Design review of the part built by this model. Coordinates are the model's own, in mm. A direction names the side the tool comes from. Give positions to 0.01 mm unless a question says otherwise; leave off trailing zeros. Loops run counter-clockwise (first coordinate to the right, second up) from the corner with the lowest first, then second, coordinate; pieces in that order, holes last.
Autodesk Inventor part; units mm, degrees
ref_plane "YZ Plane" through (0, 0, 0) normal (1, 0, 0) x (0, 1, 0)
ref_plane "XZ Plane" through (0, 0, 0) normal (0, 1, 0) x (-1, 0, 0)
ref_plane "XY Plane" through (0, 0, 0) normal (0, 0, 1) x (1, 0, 0)
sketch "Esboço1" plane through (0, 0, 0) normal (0, 1, 0) x (-1, 0, 0)
  line L0 (-70, 60) -> (70, 60)
  line L1 (70, 60) -> (70, -60)
  line L2 (70, -60) -> (-70, -60)
  line L3 (-70, -60) -> (-70, 60)
  line L4 (-70, 60) -> (70, -60) construction
  line L5 (70, 60) -> (-70, -60) construction
  point P0 (0, 0)
  dimension "d0" = 140
  dimension "d1" = 120
extrude "Extrusão1" add sketch "Esboço1" along normal blind 1.6
sketch "Esboço2" plane through (0, 1.6, 0) normal (0, 1, 0) x (1, 0, 0)
  line L0 (-94.6357, 0) -> (83.6022, 0)
  line L1 (-70, -37) -> (-52, -37)
  line L2 (-52, 37) -> (-70, 37)
  line L3 (-70, 37) -> (-70, -37)
  line L4 (-70, -37) -> (-52, 37) construction
  line L5 (-52, -37) -> (-70, 37) construction
  line L6 (-70, 60) -> (-70, -60)
  line L7 (-70, 0) -> (-70, 0)
  line L8 (-70, 0) -> (-25, 0)
  circle A0 centre (-25, 0) radius 12.5
  line L9 (-70, -60) -> (70, -60)
  line L10 (-20, -60) -> (-50, -60)
  line L11 (-20, -60) -> (10, -60)
  line L12 (70, 60) -> (-70, 60)
  line L13 (-55, -60) -> (5, -60)
  line L14 (5, -60) -> (5, -45)
  line L15 (-55, -45) -> (-55, -60)
  line L16 (-52, 0) -> (-70, 0)
  line L17 (-56, 25) -> (-48, 25)
  line L18 (-48, 25) -> (-48, -25)
  line L19 (-48, -25) -> (-56, -25)
  line L20 (-56, -25) -> (-56, 25)
  line L21 (-56, 25) -> (-48, -25) construction
  line L22 (-48, 25) -> (-56, -25) construction
  line L23 (-55, 60) -> (5, 60)
  line L24 (5, 60) -> (5, 45)
  line L25 (-55, 45) -> (-55, 60)
  line L26 (-25, 76.0053) -> (-25, -77.5323)
  line L27 (-35, -45) -> (-35, -37)
  line L28 (-35, -37) -> (-15, -37)
  line L29 (-15, -37) -> (-15, -45)
  line L30 (5, -45) -> (-15, -45)
  line L31 (-35, -45) -> (-55, -45)
  line L32 (-35, 45) -> (-35, 37)
  line L33 (-35, 37) -> (-15, 37)
  line L34 (-15, 37) -> (-15, 45)
  line L35 (5, 45) -> (-15, 45)
  line L36 (-35, 45) -> (-55, 45)
  line L37 (-55, -60) -> (5, -45) construction
  line L38 (5, -60) -> (-55, -45) construction
  line L39 (-35, 45) -> (-15, 37) construction
  line L40 (-15, 45) -> (-35, 37) construction
  point P0 (0, 0)
  point P1 (-61, 0)
  point P2 (-25, 41)
  dimension "d4" = 18
  dimension "d5" = 74
  dimension "d6" = 0
  dimension "d7" = 45
  dimension "d8" = 25
  dimension "d28" = 15
  dimension "d30" = 18
  dimension "d31" = 8
  dimension "d32" = 50
  dimension "d35" = 15
  dimension "d36" = 20
  dimension "d38" = 8
  dimension "d40" = 20
  dimension "d41" = 8
  dimension "d42" = 60
  dimension "d43" = 60
extrude "Extrusão4" cut sketch "Esboço2" against normal through all contours L26 A0 L0 | L26 A0 L0 | L0 A0 L26 | L0 A0 L26 | L18 L19 L20 L0 | L0 L20 L17 L18
sketch "Esboço3" plane through (0, 1.6, 0) normal (0, 1, 0) x (1, 0, 0)
  line L0 (44.5, -40) -> (30, -40) construction
  line L1 (30, -40) -> (30, -72.5) construction
  line L2 (30, -72.5) -> (44.5, -72.5) construction
  line L3 (44.5, -72.5) -> (44.5, -40) construction
  line L4 (30, 40) -> (44.5, 40) construction
  line L5 (44.5, 40) -> (44.5, 72.5) construction
  line L6 (44.5, 72.5) -> (30, 72.5) construction
  line L7 (30, 72.5) -> (30, 40) construction
  line L8 (37.25, -40) -> (37.25, -47.2) construction
  circle A0 centre (37.25, -47.2) radius 1.5
  line L9 (37.25, 40) -> (37.25, 47.2) construction
  circle A1 centre (37.25, 47.2) radius 1.5
  line L10 (-70, 60) -> (-70, -60)
  line L11 (52, 14) -> (49.5, 14) construction
  line L12 (49.5, 14) -> (49.5, -14) construction
  line L13 (49.5, -14) -> (52, -14) construction
  line L14 (52, -14) -> (52, 14) construction
  line L15 (52, 14) -> (49.5, -14) construction
  line L16 (49.5, 14) -> (52, -14) construction
  line L17 (54, 16) -> (47.5, 16)
  line L18 (47.5, 16) -> (47.5, -16) construction
  line L19 (47.5, -16) -> (54, -16) construction
  line L20 (54, -16) -> (54, 16)
  line L21 (70, -60) -> (70, 60)
  line L22 (5, -54.0532) -> (28, -36.1915)
  line L23 (28, -36.1915) -> (28, -58)
  line L24 (44.5, -69.5) -> (44.5446, -69.5)
  line L25 (46.5, -58) -> (46.5, -38)
  line L26 (46.5, -38) -> (46.5, -36.8245)
  line L27 (46.5, -58) -> (28, -58)
  line L28 (-70, -60) -> (70, -60)
  line L29 (7, -60) -> (5, -60)
  line L30 (70, 60) -> (-70, 60)
  line L31 (70, 60) -> (7, 60)
  line L32 (5, 54.0532) -> (28, 36.1915)
  line L33 (28, 58) -> (28, 36.1915)
  line L34 (44.5446, 69.5) -> (44.5, 69.5)
  line L35 (46.5, 58) -> (28, 58)
  line L36 (46.5, 36.8245) -> (46.5, 58)
  line L37 (5, 54.0532) -> (5, 60)
  line L38 (5, -54.0532) -> (5, -60)
  line L39 (54, -16) -> (54, -31)
  line L40 (54, -31) -> (46.5, -36.8245)
  line L41 (54, 16) -> (54, 31)
  line L42 (54, 31) -> (46.5, 36.8245)
  point P0 (0, 0)
  dimension "d59" = 14.5
  dimension "d60" = 32.5
  dimension "d63" = 32.5
  dimension "d64" = 14.5
  dimension "d76" = 7.2
  dimension "d77" = 3
  dimension "d78" = 7.2
  dimension "d79" = 3
  dimension "d97" = 2.5
  dimension "d98" = 28
  dimension "d99" = 2
  dimension "d103" = 2
  dimension "d104" = 2
  dimension "d105" = 63
  dimension "d107" = 2
  dimension "d132" = 15
  dimension "d133" = 15
sketch "Esboço4" plane through (0, 1.6, 0) normal (0, 1, 0) x (1, 0, 0)
  line L0 (-70, 60) -> (-70, -60)
  line L1 (-70, 0) -> (-70, -100)
  line L2 (-70, -100) -> (180, -100)
  line L3 (180, -100) -> (180, 100)
  line L4 (180, 100) -> (-70, 100)
  line L5 (-70, 100) -> (-70, -100)
  line L6 (250, 0) -> (-150, 0)
  line L7 (-430, 10) -> (570, 10)
  line L8 (570, 10) -> (570, -10)
  line L9 (570, -10) -> (-430, -10)
  line L10 (-430, -10) -> (-430, 10)
  line L11 (70, -60) -> (70, 60)
  line L12 (-430, 10) -> (570, -10) construction
  line L13 (570, 10) -> (-430, -10) construction
  line L14 (27.5, -90) -> (47.5, -90)
  line L15 (47.5, -90) -> (47.5, -50)
  line L16 (47.5, -50) -> (27.5, -50)
  line L17 (27.5, -50) -> (27.5, -90)
  line L18 (27.5, -90) -> (47.5, -50) construction
  line L19 (47.5, -90) -> (27.5, -50) construction
  line L20 (70, 60) -> (-70, 60)
  line L21 (47.5, 90) -> (27.5, 90)
  line L22 (27.5, 90) -> (27.5, 50)
  line L23 (27.5, 50) -> (47.5, 50)
  line L24 (47.5, 50) -> (47.5, 90)
  line L25 (47.5, 90) -> (27.5, 50) construction
  line L26 (27.5, 90) -> (47.5, 50) construction
  line L27 (0, -100) -> (0, 100) construction
  point P0 (0, 0)
  point P1 (70, 0)
  point P2 (37.5, -70)
  point P3 (37.5, 70)
  dimension "d53" = 100
  dimension "d54" = 250
  dimension "d55" = 200
  dimension "d65" = 1000
  dimension "d66" = 20
  dimension "d68" = 20
  dimension "d69" = 40
  dimension "d70" = 20
  dimension "d71" = 40
  dimension "d72" = 40
  dimension "d73" = 40
  dimension "d80" = 37.5
  dimension "d81" = 37.5
extrude "Extrusão5" cut sketch "Esboço3" against normal through all contours A0 | A1
sketch "Esboço5" plane through (0, 1.6, 0) normal (0, 1, 0) x (1, 0, 0)
  line L0 (70, 60) -> (-70, 60)
  line L1 (-70, 60) -> (-55, 60)
  line L2 (-55, 60) -> (-55, 39)
  line L3 (-55, 39) -> (-70, 39)
  line L4 (-70, 39) -> (-70, 60)
  line L5 (-70, -60) -> (70, -60)
  line L6 (-70, -60) -> (-55, -60)
  line L7 (-55, -60) -> (-55, -39)
  line L8 (-55, -39) -> (-70, -39)
  line L9 (-70, -39) -> (-70, -60)
  line L10 (-70, 60) -> (-70, -60)
  line L11 (-55, 39) -> (-70, 39)
  line L12 (-70, 39) -> (-70, 60)
  line L13 (-70, 60) -> (-55, 60)
  line L14 (-55, 60) -> (-55, 39)
  line L15 (-55, -39) -> (-70, -39)
  line L16 (-70, -39) -> (-70, -60)
  line L17 (-70, -60) -> (-55, -60)
  line L18 (-55, -60) -> (-55, -39)
  point P0 (0, 0)
  dimension "d84" = 15
  dimension "d85" = 21
  dimension "d86" = 15
  dimension "d87" = 21
extrude "Extrusão6" cut sketch "Esboço5" against normal through all
fillet "Arredondamento1" radius 2 10 edges at (-70, 0.8, 39) (-55, 0.8, 39) (-55, 0.8, 60) (-56, 0.8, 25) (-48, 0.8, 25) (-56, 0.8, -25) (-48, 0.8, -25) (-70, 0.8, -39) (-55, 0.8, -39) (-55, 0.8, -60)
sketch "Esboço7" plane through (0, 1.6, 0) normal (0, 1, 0) x (1, 0, 0)
  line L0 (-3.4695, -17.196) -> (-3.4695, -2.1961) construction
  line L1 (-3.4695, -2.1961) -> (11.6526, -2.1961) construction
  line L2 (11.6526, -2.1961) -> (11.6526, -17.196) construction
  line L3 (11.6526, -17.196) -> (-3.4695, -17.196) construction
  point P0 (0, 0)
extrude "Extrusão10" cut sketch "Esboço3" against normal through all contours L30 L21 L28 L38 L22 L23 L27 L25 L26 L40 L39 L20 L41 L42 L36 L35 L33 L32 L37
fillet "Arredondamento4" radius 2 14 edges at (5, 0.8, 60) (5, 0.8, 54.0532) (28, 0.8, 36.1915) (28, 0.8, 58) (46.5, 0.8, 58) (46.5, 0.8, 36.8245) (54, 0.8, 31) (54, 0.8, -31) (46.5, 0.8, -36.8245) (46.5, 0.8, -58) (28, 0.8, -58) (28, 0.8, -36.1915) (5, 0.8, -54.0532) (5, 0.8, -60)
sketch "Esboço8" plane through (0, 1.6, 0) normal (0, 1, 0) x (1, 0, 0)
  line L0 (-55, -60) -> (5, -60)
  line L1 (5, -60) -> (5, -50)
  line L2 (5, -50) -> (-55, -50)
  line L3 (-55, -50) -> (-55, -60)
  circle A0 centre (-51.25, -55) radius 1.5
  circle A1 centre (1.25, -55) radius 1.5
  line L4 (-70, 37) -> (-70, -37)
  line L5 (-70, 0) -> (54, 0)
  line L6 (54, 30.0209) -> (54, -30.0209)
  line L7 (-55, 60) -> (5, 60)
  line L8 (5, 60) -> (5, 50)
  line L9 (5, 50) -> (-55, 50)
  line L10 (-55, 50) -> (-55, 60)
  circle A2 centre (-51.25, 55) radius 1.5
  circle A3 centre (1.25, 55) radius 1.5
  point P0 (0, 0)
  point P1 (-55, -55)
  dimension "d137" = 60
  dimension "d138" = 10
  dimension "d140" = 3
  dimension "d142" = 3
  dimension "d143" = 3.75
  dimension "d144" = 3.75
  dimension "d145" = 5
  dimension "d146" = 5
  dimension "d147" = 60
  dimension "d148" = 10
  dimension "d149" = 3
  dimension "d150" = 3
  dimension "d151" = 3.75
  dimension "d152" = 5
  dimension "d153" = 5
  dimension "d154" = 3.75
extrude "Extrusão11" cut sketch "Esboço8" against normal through all contours A0 | A1 | A2 | A3
sketch "Esboço9" plane through (0, 1.6, 0) normal (0, 1, 0) x (1, 0, 0)
  line L0 (54, -38.06) -> (50.5, -38.06)
  line L1 (50.5, -38.06) -> (50.5, 41.775)
  line L2 (50.5, 41.775) -> (54, 41.775)
  line L3 (54, 41.775) -> (54, -38.06)
  line L4 (52.2999, -27) -> (48.7001, -27)
  line L5 (48.7001, -27) -> (48.7001, 27)
  line L6 (48.7001, 27) -> (52.2999, 27)
  line L7 (52.2999, 27) -> (52.2999, -27)
  line L8 (52.2999, -27) -> (48.7001, 27) construction
  line L9 (48.7001, -27) -> (52.2999, 27) construction
  circle A0 centre (50.5, -27) radius 1.5
  circle A1 centre (50.5, 27) radius 1.5
  point P0 (0, 0)
  point P1 (50.5, 0)
  dimension "d158" = 3.5
  dimension "d159" = 54
  dimension "d160" = 3
  dimension "d161" = 3
extrude "Extrusão12" cut sketch "Esboço9" against normal through all contours A0 L4 L1 | L1 L4 A0 | L4 A0 L1 | L1 A0 L4 | A1 L6 L1 | L1 L6 A1 | L6 A1 L1 | L1 A1 L6
properties part number "PCB"
Q1. Take a section at B-B (z = 47.2). Give the boundary of the cut face in (x, y).
Results:
outline: (-55, 0) - (13.82, 0) - (13.82, 1.6) - (-55, 1.6) - close; (28, 0) - (35.75, 0) - (35.75, 1.6) - (28, 1.6) - close; (38.75, 0) - (46.5, 0) - (46.5, 1.6) - (38.75, 1.6) - close
Q2. Take a section at C-C (x = -18). Give the boundary of the cut face in (y, z), plus the area to 3 significant figures.
Results:
outline: (0, -60) - (1.6, -60) - (1.6, -10.36) - (0, -10.36) - close; (0, 10.36) - (1.6, 10.36) - (1.6, 60) - (0, 60) - close
area: 159 mm2
Q3. Insertion check: pin 1 (1.5 mm diameter, centred on x = -50, z = 12.5, fed in from -Y); pin 2 (8 mm diameter, centred on x = -44.5, z = -5.5, fed in from -Y); pin 3 (0.8 mm diameter, centred on y = 1, z = -56, fed in from +X); pin 4 (0.5 mm diameter, centred on x = -60, y = 1, fed in from -Z). Each pin has a flat end and moves straight along its axis. Give the tip position at first contact, or say it passes through.
Results:
pin 1: passes through
pin 2: stops at y = 0
pin 3: stops at x = 46.5
pin 4: stops at z = -39
Q4. Tool access review of faces 5 (the face through (15.14, 0.81, 46.18)), 6 (the face through (15.14, 0.81, -46.18)), 7 (the face through (-34.92, 0.811, 7.606)): name each direction out of +Z, -Z, +X, -X, +Y, -Y from which nothing blocks a thin tool from reaching the whole face with its end or side.
Results:
face 5: +Z, +Y, -Y
face 6: -Z, +Y, -Y
face 7: +Y, -Y
Q5. Wall thickness on line 1 (Z direction, x = -51.25, y = 0.5); line 2 (X direction, y = 1.25, z = 55); line 3 (X direction, y = 0.95, z = 0): over which ranges is each line inside the solid? List them lowest first.
Results:
line 1: z = -60 to -56.5, -53.5 to -25, 25 to 53.5, 56.5 to 60
line 2: x = -55 to -52.75, -49.75 to -0.25, 2.75 to 5, 28 to 46.5
line 3: x = -70 to -56, -48 to -37.5, -12.5 to 54
Q6. Take a section at A-A (x = 37.25). Give the boundary of the cut face in (y, z), plus the area to 3 significant figures.
Results:
outline: (0, -58) - (1.6, -58) - (1.6, -48.7) - (0, -48.7) - close; (0, -45.7) - (1.6, -45.7) - (1.6, 45.7) - (0, 45.7) - close; (0, 48.7) - (1.6, 48.7) - (1.6, 58) - (0, 58) - close
area: 176 mm2
Q7. Draft analysis for pull direction X (two halves, no side actions). For faces 1 (the face through (36.06, 0.81, 48.11)), 2 (the face through (50.29, 0.81, -33.88)), 3 (the face through (-52.44, 0.81, 55.91)), 4 (the face through (-7, 1.6, 1)), state which applies: pulls with the +X half, pulls with the -X half, needs draft (parallel to the pull), parting line crosses it, or undercut.
Results:
face 1: undercut
face 2: pulls with the +X half
face 3: undercut
face 4: needs draft
Q8. Take a section at D-D (y = 0.3). Give the number of separate pieces and of enclosed holes in the cut face, plus the area to 3 significant figures.
Results:
separate pieces: 1
enclosed holes: 10
area: 12,200 mm2
